```python
from build123d import *

# Parameters (mm, degrees)
SKETCH1_R           = 7.5
BOSS_EXTRUDE1_DEPTH = 1
SKETCH4_R           = 6
BOSS_EXTRUDE2_DEPTH = 4.6
SKETCH5_R           = 4.95
CUT_EXTRUDE1_DEPTH  = 5.6


with BuildPart() as part:
    # Sketch1 → Boss-Extrude1 (new body)
    with BuildSketch(Plane(origin=(0, 0, 0), x_dir=(1, 0, 0), z_dir=(0, 1, 0))):
        Circle(SKETCH1_R)
    extrude(amount=BOSS_EXTRUDE1_DEPTH)

    # Sketch2 one side → Revolve1 (revolve)
    with BuildSketch(Plane.XY):
        with BuildLine():
            Line((0, 1), (7.5, 1))
            ThreePointArc((7.5, 1), (3.829246009, 2.158448432), (0, 2.55))
            Line((0, 2.55), (0, 1))
        make_face()
    revolve(axis=Axis((0, 2.55, 0), (0, -1, 0)))

    # Sketch4 → Boss-Extrude2 (add)
    with BuildSketch(Plane.XZ):
        Circle(SKETCH4_R)
    extrude(amount=BOSS_EXTRUDE2_DEPTH)

    # Sketch5 → Cut-Extrude1 (cut)
    with BuildSketch(Plane.XZ.offset(4.6)):
        Circle(SKETCH5_R)
    extrude(amount=-CUT_EXTRUDE1_DEPTH, mode=Mode.SUBTRACT)


solid = part.part
```
Verification items for the finished model (mm, model axes). A direction names the side the tool comes from. Coordinates: 2 decimals unless noted, no trailing zeros. Loops run counter-clockwise (first coordinate to the right, second up) from the corner with the lowest first, then second, coordinate; pieces in that order, holes last. Notation, with made-up numbers: (-30, -7) - (9, -7) arc R24 cw to (9, 12) - close; hole circle Ø8 at (73.25, 83). An arc over 180 degrees is marked (long way). Put each result on its own line as item: value.
Item 1: Section check C-C (y = -2). Enter the section's corners in (x, z), then the cut area to 3 significant figures.
Conclusion:
outline: circle Ø12 at (0, 0); hole circle Ø9.9 at (0, 0)
area: 36.1 mm2
Item 2: Section check A-A (x = 0). Enter the section's corners in (y, z).
Conclusion:
outline: (-4.6, -6) - (0, -6) - (0, -7.5) - (1, -7.5) arc R18.92 ccw to (1, 7.5) - (0, 7.5) - (0, 6) - (-4.6, 6) - (-4.6, 4.95) - (1, 4.95) - (1, -4.95) - (-4.6, -4.95) - close
Item 3: Draft check along X on faces 1 (the face through (-6, -2, 0)), 2 (the face through (0, 1, 0)), 3 (the face through (4.72, -1.84, 1.49)), 4 (the face through (-1.36, -4.6, 4.92)). Enter one of: pulls with the +X half, pulls with the -X half, needs draft (parallel to the pull), parting line crosses it, or undercut.
Conclusion:
face 1: parting line crosses it
face 2: undercut
face 3: undercut
face 4: needs draft
Item 4: Section check B-B (z = 0). Enter the section's corners in (x, y), then the cut area to 3 significant figures.
Conclusion:
outline: (-7.5, 0) - (-6, 0) - (-6, -4.6) - (-4.95, -4.6) - (-4.95, 1) - (4.95, 1) - (4.95, -4.6) - (6, -4.6) - (6, 0) - (7.5, 0) - (7.5, 1) arc R18.92 ccw to (-7.5, 1) - close
area: 30.4 mm2
Item 5: Gauge pin test, flat ends, axial feed: pin 1 Ø1.5 at (y, z) = (-3.5, -2.5) entering from +X; pin 2 Ø1.5 at (y, z) = (0.5, -1) entering from -X; pin 3 Ø4 at (x, y) = (5.5, -1.5) entering from -Z. Record the tip position at first contact, or that the pin passes through.
Conclusion:
pin 1: stops at x = 5.74
pin 2: stops at x = -7.5
pin 3: stops at z = -6.23
Item 6: Set-up check for faces 5 (the face through (2, 0, -6)), 6 (the face through (-7.493, 0.493, -0.33)): record each of +Z, -Z, +X, -X, +Y, -Y from which the full face is reachable in a straight line by a thin tool's end or side.
Conclusion:
face 5: -Y
face 6: +Y, -Y
Item 7: Section check D-D (y = 1.75). Enter the section's corners in (x, z).
Conclusion:
outline: circle Ø10.89 at (0, 0)
Item 8: Scan lines: line 1 along Z through (x, y) = (0, -1.65); line 2 along X through (y, z) = (-1.25, -3.5); line 3 along X through (y, z) = (-3.5, 1.75). Record each from-to range of solid material in increasing order.
Conclusion:
line 1: z = -6 to -4.95, 4.95 to 6
line 2: x = -4.87 to -3.5, 3.5 to 4.87
line 3: x = -5.74 to -4.63, 4.63 to 5.74
